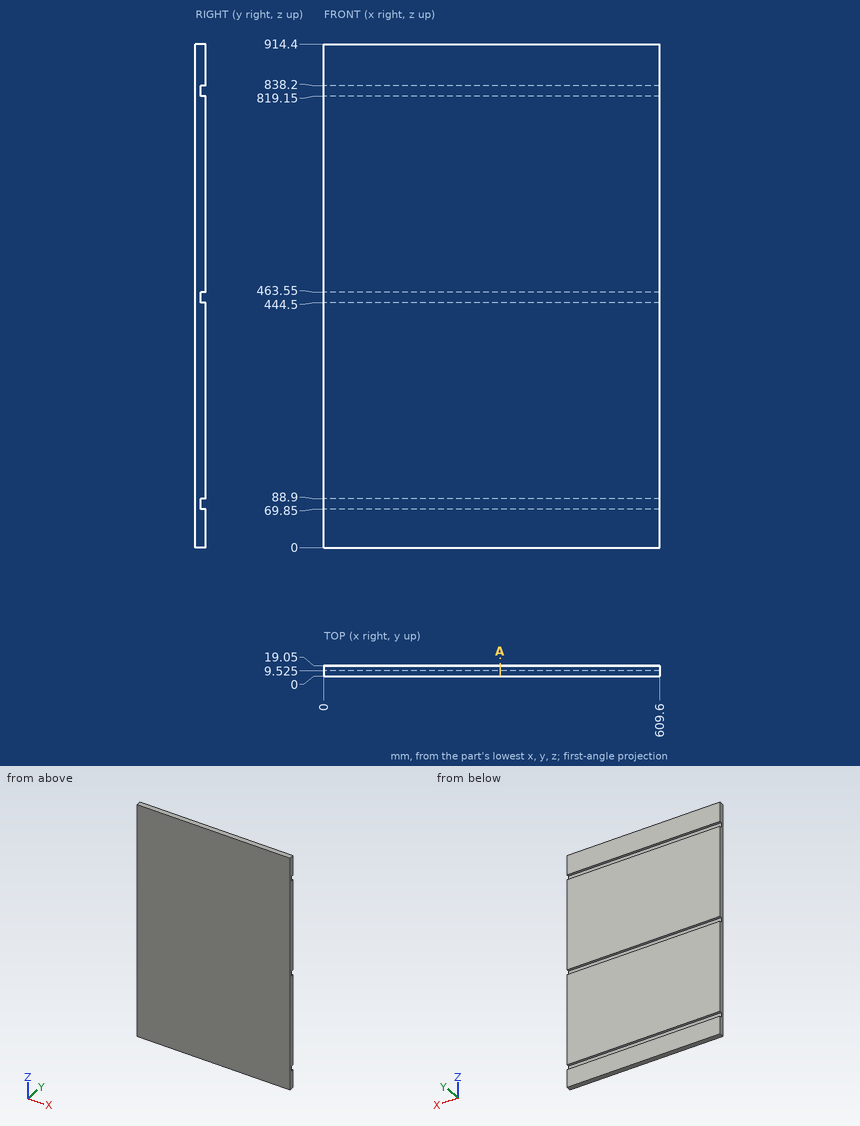
Design review of the part shown in the three views and the two pictorial views. Dimensions are in mm from the part's minimum x, y and z. Give positions to 0.01 mm unless a question says otherwise; leave off trailing zeros. Loops run counter-clockwise (first coordinate to the right, second up) from the corner with the lowest first, then second, coordinate; pieces in that order, holes last. Notation, with made-up numbers: M 33,-7 L 91,-7 A16 ccw 91,22 Z; hole C 59,6 d10. An arc over 180 degrees is marked long. Put each result on its own line as item: value. Start each with the question number.
(1) For pin 1 (7.5 mm diameter, centred on x = 299, y = 13, fed in from -Z); pin 2 (5.5 mm diameter, centred on x = 382.5, z = 453.5, fed in from +Y) (3 decimals), all flat-tipped, find the tip position at first contact; note any pin that passes through.
(2) Wall thickness on L1, parallel to Z at x = 323, y = 13.75: over which ranges is the line inside the solid? List them lowest first.
(3) Add section A-A, the plane x = 320. Write out the cut boundary in (y, z) (3 decimals), then the cut area to 3 significant figures.
Result:
1. pin 1: stops at z = 0
1. pin 2: stops at y = 9.525
2. L1: z = 0 to 69.85, 88.9 to 444.5, 463.55 to 819.15, 838.2 to 914.4
3. outline: M 0,0 L 19.05,0 L 19.05,69.85 L 9.525,69.85 L 9.525,88.9 L 19.05,88.9 L 19.05,444.5 L 9.525,444.5 L 9.525,463.55 L 19.05,463.55 L 19.05,819.15 L 9.525,819.15 L 9.525,838.2 L 19.05,838.2 L 19.05,914.4 L 0,914.4 Z
3. area: 16,900 mm^2
